from build123d import *
from OCP.BRepFilletAPI import BRepFilletAPI_MakeChamfer

# Parameters (mm, degrees)
ESBO_O1_R                 = 4.5
RESSALTO_EXTRUS_O1_DEPTH  = 3
ESBO_O2_R                 = 4.5
RESSALTO_EXTRUS_O2_DEPTH  = 3
CHANFRO1_SIZE             = 4
CHANFRO1_SIZE_2           = 3
FURO_ROSCADO_DE_M3X0_51_D = 2.5
ESBO_O6_R                 = 4.5
ESBO_O6_R_2               = 3.75
RESSALTO_EXTRUS_O3_DEPTH  = 3
CORTE_EXTRUS_O1_REACH     = 51.391
ESBO_O7_R                 = 1.5
CORTE_EXTRUS_O2_REACH     = 51.391
ESBO_O8_R                 = 1.5
CHANFRO2_SIZE             = 0.75
CORTE_EXTRUS_O4_REACH     = 51.391
ESBO_O14_R                = 2.5
CHANFRO3_SIZE             = 0.5
ESBO_O15_R                = 1.9
CORTE_EXTRUS_O5_DEPTH     = 1


# Some blends are built 0.0001 mm under size
with BuildPart() as part:
    # Esboço1 → Ressalto-extrusão1 (new body)
    with BuildSketch(Plane.XY):
        with BuildLine():
            Line((-6, 6), (-6, 39))
            Line((-6, 39), (-6, 40))
            ThreePointArc((-6, 40), (-4.535533906, 43.535533906), (-1, 45))
            Line((-1, 45), (17.98112418, 45))
            Line((17.98112418, 45), (19.454538911, 33))
            Line((19.454538911, 33), (17.98112418, 33))
            Line((17.98112418, 33), (6, 33))
            Line((6, 33), (6, 25))
            Line((6, 25), (6, 6))
            ThreePointArc((6, 6), (4.242640687, 1.757359313), (0, 0))
            ThreePointArc((0, 0), (-4.242640687, 1.757359313), (-6, 6))
        make_face()
        with Locations((0, 39)):
            Circle(ESBO_O1_R, mode=Mode.SUBTRACT)
    extrude(amount=RESSALTO_EXTRUS_O1_DEPTH)

    # Esboço2 → Ressalto-extrusão2 (add)
    with BuildSketch(Plane.XY.offset(3)):
        with BuildLine():
            Line((6, 25), (6, 18))
            Line((6, 18), (1.171572875, 13.171572875))
            ThreePointArc((1.171572875, 13.171572875), (-0.12612052, 12.30448187), (-1.656854249, 12))
            Line((-1.656854249, 12), (-6, 12))
            Line((-6, 12), (-6, 25))
            Line((-6, 25), (-6, 40))
            ThreePointArc((-6, 40), (-4.535533906, 43.535533906), (-1, 45))
            Line((-1, 45), (17.98112418, 45))
            Line((17.98112418, 45), (19.454538911, 33))
            Line((19.454538911, 33), (6, 33))
            Line((6, 33), (6, 25))
        make_face()
        with Locations((0, 39)):
            Circle(ESBO_O2_R, mode=Mode.SUBTRACT)
    extrude(amount=RESSALTO_EXTRUS_O2_DEPTH)

    # Chanfro1
    chanfro1_edges_1 = [part.edges().sort_by_distance(p)[0] for p in [
        (3.585786438, 15.585786438, 6),
    ]]
    chanfro1_side_1 = [part.faces().sort_by_distance(p)[0] for p in [
        (3.543360031, 15.628212844, 6),
    ]]
    chanfro1_edges_2 = [part.edges().sort_by_distance(p)[0] for p in [
        (-0.12612052, 12.30448187, 6),
    ]]
    chanfro1_side_2 = [part.faces().sort_by_distance(p)[0] for p in [
        (-0.149081526, 12.359914642, 6),
    ]]
    chanfro1_edges_3 = [part.edges().sort_by_distance(p)[0] for p in [
        (-3.828427125, 12, 6),
    ]]
    chanfro1_side_3 = [part.faces().sort_by_distance(p)[0] for p in [
        (-3.828427125, 12, 5.94),
    ]]
    chanfro1 = BRepFilletAPI_MakeChamfer(part.part.solid().wrapped)
    for e in chanfro1_edges_1:
        chanfro1.Add(CHANFRO1_SIZE - 0.0001, CHANFRO1_SIZE_2 - 0.0001, e.wrapped, chanfro1_side_1[0].wrapped)
    for e in chanfro1_edges_2:
        chanfro1.Add(CHANFRO1_SIZE - 0.0001, CHANFRO1_SIZE_2 - 0.0001, e.wrapped, chanfro1_side_2[0].wrapped)
    for e in chanfro1_edges_3:
        chanfro1.Add(CHANFRO1_SIZE_2 - 0.0001, CHANFRO1_SIZE - 0.0001, e.wrapped, chanfro1_side_3[0].wrapped)
    add(Compound.cast(chanfro1.Shape()), mode=Mode.REPLACE)  # a hair under: the kernel refuses the full size

    # Furo roscado de M3x0.51 (through all)
    with Locations(Plane(origin=(0, 45, 0), x_dir=(1, 0, 0), z_dir=(0, 1, 0))):
        with Locations((8, -3)):
            Hole(FURO_ROSCADO_DE_M3X0_51_D / 2)

    # Esboço6 → Ressalto-extrusão3 (add)
    with BuildSketch(Plane(origin=(0, 0, 0), x_dir=(-1, 0, 0), z_dir=(0, 0, -1))):
        with Locations((0, 39)):
            Circle(ESBO_O6_R)
        with Locations((0, 39)):
            Circle(ESBO_O6_R_2, mode=Mode.SUBTRACT)
    extrude(amount=-RESSALTO_EXTRUS_O3_DEPTH)

    # Esboço7 → Corte-extrusão1 (cut, up to next)
    with BuildSketch(Plane(origin=(0, 0, 0), x_dir=(-1, 0, 0), z_dir=(0, 0, -1)), mode=Mode.PRIVATE) as corte_extrus_o1_sk1:
        with Locations((-14.954538911, 42)):
            Circle(ESBO_O7_R)
    corte_extrus_o1_tool1 = extrude(corte_extrus_o1_sk1.sketch, amount=-CORTE_EXTRUS_O1_REACH, mode=Mode.PRIVATE) & part.part
    # Esboço7 → Corte-extrusão1 (cut, up to next)
    with BuildSketch(Plane(origin=(0, 0, 0), x_dir=(-1, 0, 0), z_dir=(0, 0, -1)), mode=Mode.PRIVATE) as corte_extrus_o1_sk2:
        with Locations((-14.954538911, 36)):
            Circle(ESBO_O7_R)
    corte_extrus_o1_tool2 = extrude(corte_extrus_o1_sk2.sketch, amount=-CORTE_EXTRUS_O1_REACH, mode=Mode.PRIVATE) & part.part
    add(corte_extrus_o1_tool1.solids().sort_by_distance((14.954539, 42, 0))[0], mode=Mode.SUBTRACT)
    add(corte_extrus_o1_tool2.solids().sort_by_distance((14.954539, 36, 0))[0], mode=Mode.SUBTRACT)

    # Esboço8 → Corte-extrusão2 (cut, up to next)
    with BuildSketch(Plane.XY.offset(6), mode=Mode.PRIVATE) as corte_extrus_o2_sk1:
        with Locations((2.171572875, 24)):
            Circle(ESBO_O8_R)
    corte_extrus_o2_tool1 = extrude(corte_extrus_o2_sk1.sketch, amount=-CORTE_EXTRUS_O2_REACH, mode=Mode.PRIVATE) & part.part
    # Esboço8 → Corte-extrusão2 (cut, up to next)
    with BuildSketch(Plane.XY.offset(6), mode=Mode.PRIVATE) as corte_extrus_o2_sk2:
        with Locations((-3.828427125, 18)):
            Circle(ESBO_O8_R)
    corte_extrus_o2_tool2 = extrude(corte_extrus_o2_sk2.sketch, amount=-CORTE_EXTRUS_O2_REACH, mode=Mode.PRIVATE) & part.part
    add(corte_extrus_o2_tool1.solids().sort_by_distance((2.171573, 24, 6))[0], mode=Mode.SUBTRACT)
    add(corte_extrus_o2_tool2.solids().sort_by_distance((-3.828427, 18, 6))[0], mode=Mode.SUBTRACT)

    # Chanfro2
    # the kernel refuses this chamfer: 0.75 mm, written as the material it takes off along each edge
    with BuildSketch(Plane(origin=(2.171572875, 24, 6), x_dir=(1, 0, 0), z_dir=(0, -1, 0))) as chanfro2_piece_1:
        Polygon((1.5 + CHANFRO2_SIZE, 0), (1.5, -CHANFRO2_SIZE), (1.5, 0), align=None)
    revolve(axis=Axis((2.171572875, 24, 6), (0, 0, 1)), mode=Mode.SUBTRACT)
    with BuildSketch(Plane(origin=(-3.828427125, 18, 6), x_dir=(1, 0, 0), z_dir=(0, -1, 0))) as chanfro2_piece_2:
        Polygon((1.5 + CHANFRO2_SIZE, 0), (1.5, -CHANFRO2_SIZE), (1.5, 0), align=None)
    revolve(axis=Axis((-3.828427125, 18, 6), (0, 0, 1)), mode=Mode.SUBTRACT)

    # Esboço14 → Corte-extrusão4 (cut, up to next)
    with BuildSketch(Plane(origin=(0, 0, 0), x_dir=(-1, 0, 0), z_dir=(0, 0, -1)), mode=Mode.PRIVATE) as corte_extrus_o4_sk1:
        with Locations((0, 6)):
            Circle(ESBO_O14_R)
    corte_extrus_o4_tool1 = extrude(corte_extrus_o4_sk1.sketch, amount=-CORTE_EXTRUS_O4_REACH, mode=Mode.PRIVATE) & part.part
    add(corte_extrus_o4_tool1.solids().sort_by_distance((0, 6, 0))[0], mode=Mode.SUBTRACT)

    # Chanfro3
    chanfro3_edges = [part.edges().sort_by_distance(p)[0] for p in [
        (2.5, 6, 3),
    ]]
    chamfer(chanfro3_edges, length=CHANFRO3_SIZE)

    # Esboço15 → Corte-extrusão5 (cut)
    with BuildSketch(Plane(origin=(0, 0, 0), x_dir=(-1, 0, 0), z_dir=(0, 0, -1))):
        with Locations((-2.171572875, 24)):
            Circle(ESBO_O15_R)
        with Locations((3.828427125, 18)):
            Circle(ESBO_O15_R)
    extrude(amount=-CORTE_EXTRUS_O5_DEPTH, mode=Mode.SUBTRACT)


solid = part.part
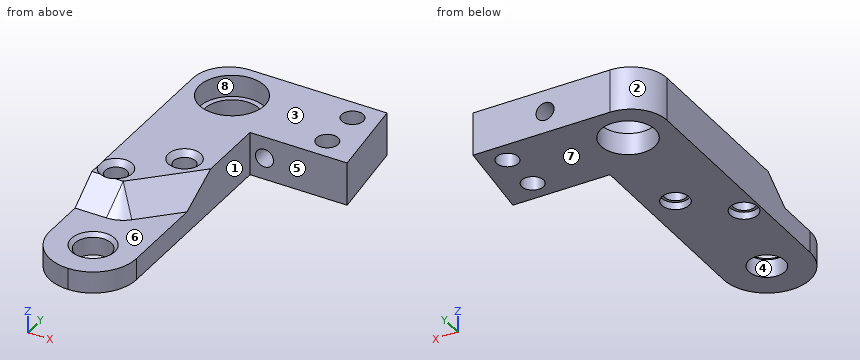
Geometry check sheet. Reference: the model listing, model coordinates, mm. Face numbers are marked on the shaded views. A direction names the side the tool comes from. Round coordinates to 2 decimals unless told otherwise and drop trailing zeros. Order: outer loops, then holes, each group sorted by start corner. A loop starts at its lowest first (then second) coordinate and runs counter-clockwise, first axis right, second up. Notation, with made-up numbers: (2.25, 13) -> (26.25, 13) arc R19 ccw to (26.25, 38) -> close; hole circle Ø11 at (-23, -37). An arc over 180 degrees is marked (long way). Use one line per item in the form item = value.
1. Cross-section at A-A, the plane x = 8.75. Enter the section's corners in (y, z).
Working result:
outline = (33, 0) -> (45, 0) -> (45, 2) -> (33, 2) -> close; (33, 4) -> (45, 4) -> (45, 6) -> (33, 6) -> close
2. Cross-section at D-D, the plane y = 34. Enter the section's corners in (x, z), plus the area to 3 significant figures.
Working result:
outline = (-6, 0) -> (19.33, 0) -> (19.33, 6) -> (-6, 6) -> close; hole circle Ø2.5 at (8, 3)
area = 147 mm^2
3. Cross-section at B-B, the plane y = 39. Enter the section's corners in (x, z), plus the area to 3 significant figures.
Working result:
outline = (-6, 0) -> (-3.75, 0) -> (-3.75, 3) -> (-4.5, 3) -> (-4.5, 6) -> (-6, 6) -> close; (3.75, 0) -> (18.72, 0) -> (18.72, 6) -> (4.5, 6) -> (4.5, 3) -> (3.75, 3) -> close; hole circle Ø2.5 at (8, 3)
area = 93.9 mm^2
4. Mould release check, pull along X, two halves, no side actions. Record for the marked faces 1, 2, 3 and 4: pulls with the +X half, pulls with the -X half, needs draft (parallel to the pull), parting line crosses it, or undercut.
Working result:
face_1 = pulls with the +X half
face_2 = pulls with the -X half
face_3 = needs draft
face_4 = undercut
5. Go/stop test with flat-tipped pins: pin 1 (13 mm diameter, centred on x = 2.5, y = 6, fed in from +Z); pin 2 (3 mm diameter, centred on x = 14.5, z = 1, fed in from -Y). Record where each tip stops, or that it passes through.
Working result:
pin_1 = 3
pin_2 = 33
6. Cross-section at C-C, the plane x = 14.5. Enter the section's corners in (y, z), plus the area to 3 significant figures.
Working result:
outline = (33, 0) -> (34.57, 0) -> (34.57, 6) -> (33, 6) -> close; (37.43, 0) -> (40.57, 0) -> (40.57, 6) -> (37.43, 6) -> close; (43.43, 0) -> (45, 0) -> (45, 6) -> (43.43, 6) -> close
area = 37.7 mm^2
7. Set-up check for the marked faces 5, 6, 7 and 8: record each of +Z, -Z, +X, -X, +Y, -Y from which the full face is reachable in a straight line by a thin tool's end or side.
Working result:
face_5 = +Z, -Z, +X, -Y
face_6 = +Z, +X, -Y
face_7 = -Z, +X, -X, +Y, -Y
face_8 = +Z
8. Scan lines: line 1 along Y through (x, z) = (15.25, 1.75); line 2 along Z through (x, y) = (0.25, 9); line 3 along Y through (x, z) = (0, 4.85). Record each from-to range of solid material in increasing order. Write a range as from..to.
Working result:
line_1 = 33..34.53, 37.47..40.53, 43.47..45
line_2 = 0..3
line_3 = 15.49..34.5, 43.5..45
